Source: CAD feature listing. Evaluate the final solid. Frame: model axes, mm. Face numbers are marked on the shaded views. A direction names the side the tool comes from. Give positions to 0.01 mm unless a question says otherwise; leave off trailing zeros. Loops run counter-clockwise (first coordinate to the right, second up) from the corner with the lowest first, then second, coordinate; pieces in that order, holes last.
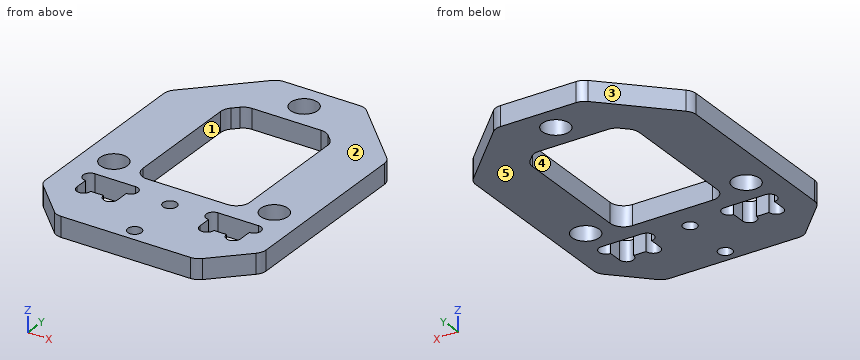
```python
from build123d import *

# Parameters (mm, degrees)
SKETCH_1_W          = 33
SKETCH_1_H          = 44.5
EXTRUDE_1_DEPTH     = 3
SKETCH_2_R          = 2.025
SKETCH_2_R_2        = 1.025
CUT_EXTRUDE_1_DEPTH = 13
CHAMFER_1_SIZE      = 10
CUT_EXTRUDE_2_DEPTH = 13
FILLET_1_R          = 2
CHAMFER_2_SIZE      = 6
FILLET_2_R          = 2
SKETCH_4_W          = 6.1
SKETCH_4_H          = 4.1
CUT_EXTRUDE_3_DEPTH = 3
SKETCH_5_R          = 1.05
CUT_EXTRUDE_4_DEPTH = 3


with BuildPart() as part:
    # 草图1 → 凸台-拉伸1 (new body)
    with BuildSketch(Plane.XY):
        Rectangle(SKETCH_1_W, SKETCH_1_H)
    extrude(amount=EXTRUDE_1_DEPTH)

    # 草图2 → 切除-拉伸1 (cut)
    with BuildSketch(Plane.XY.offset(3)):
        with Locations((12, -6.75)):
            Circle(SKETCH_2_R)
        with Locations((-12, -6.75)):
            Circle(SKETCH_2_R)
        with Locations((0, 18.25)):
            Circle(SKETCH_2_R)
        with Locations((0, -12.25)):
            Circle(SKETCH_2_R_2)
        with Locations((0, -20.25)):
            Circle(SKETCH_2_R_2)
    extrude(amount=-CUT_EXTRUDE_1_DEPTH, mode=Mode.SUBTRACT)

    # 倒角1
    chamfer_1_edges = [part.edges().sort_by_distance(p)[0] for p in [
        (-16.5, 22.25, 1.5),
        (16.5, 22.25, 1.5),
    ]]
    chamfer(chamfer_1_edges, length=CHAMFER_1_SIZE)

    # 草图3 → 切除-拉伸2 (cut)
    with BuildSketch(Plane.XY.offset(3)):
        Polygon((-8, -8.25), (8, -8.25), (8, 12.264718626), (6.014718626, 14.25), (-6.014718626, 14.25), (-8, 12.264718626), align=None)
    extrude(amount=-CUT_EXTRUDE_2_DEPTH, mode=Mode.SUBTRACT)

    # 圆角1
    fillet_1_edges = [part.edges().sort_by_distance(p)[0] for p in [
        (-8, -8.25, 1.5),
        (-8, 12.264718626, 1.5),
        (-6.014718626, 14.25, 1.5),
        (6.014718626, 14.25, 1.5),
        (8, 12.264718626, 1.5),
        (8, -8.25, 1.5),
    ]]
    fillet(fillet_1_edges, radius=FILLET_1_R)

    # 倒角2
    chamfer_2_edges = [part.edges().sort_by_distance(p)[0] for p in [
        (16.5, -22.25, 1.5),
        (-16.5, -22.25, 1.5),
    ]]
    chamfer(chamfer_2_edges, length=CHAMFER_2_SIZE)

    # 圆角2
    fillet_2_edges = [part.edges().sort_by_distance(p)[0] for p in [
        (16.5, -16.25, 1.5),
        (-10.5, -22.25, 1.5),
        (10.5, -22.25, 1.5),
        (-16.5, -16.25, 1.5),
        (-6.5, 22.25, 1.5),
        (6.5, 22.25, 1.5),
        (16.5, 12.25, 1.5),
        (-16.5, 12.25, 1.5),
    ]]
    fillet(fillet_2_edges, radius=FILLET_2_R)

    # 草图4 → 切除-拉伸3 (cut)
    with BuildSketch(Plane.XY.offset(3)):
        with Locations((-9.2, -12.75)):
            Rectangle(SKETCH_4_W, SKETCH_4_H)
        with Locations((9.2, -12.75)):
            Rectangle(SKETCH_4_W, SKETCH_4_H)
    extrude(amount=-CUT_EXTRUDE_3_DEPTH, mode=Mode.SUBTRACT)

    # 草图5 → 切除-拉伸4 (cut)
    with BuildSketch(Plane.XY.offset(3)):
        with Locations((-11.2, -14.8)):
            Circle(SKETCH_5_R)
        with Locations((-7.2, -14.8)):
            Circle(SKETCH_5_R)
        with Locations((7.2, -14.8)):
            Circle(SKETCH_5_R)
        with Locations((11.2, -14.8)):
            Circle(SKETCH_5_R)
        with Locations((-12.25, -11.75)):
            Circle(SKETCH_5_R)
        with Locations((-6.15, -11.75)):
            Circle(SKETCH_5_R)
        with Locations((6.15, -11.75)):
            Circle(SKETCH_5_R)
        with Locations((12.25, -11.75)):
            Circle(SKETCH_5_R)
    extrude(amount=-CUT_EXTRUDE_4_DEPTH, mode=Mode.SUBTRACT)


solid = part.part
```
(1) Section B-B, the plane y = -11.75. Return the cut outline in (x, z), then the cut area to 3 significant figures.
A:
outline: (-16.5, 0) - (-13.3, 0) - (-13.3, 3) - (-16.5, 3) - close; (-5.1, 0) - (-0.89, 0) - (-0.89, 3) - (-5.1, 3) - close; (0.89, 0) - (5.1, 0) - (5.1, 3) - (0.89, 3) - close; (13.3, 0) - (16.5, 0) - (16.5, 3) - (13.3, 3) - close
area: 44.4 mm2
(2) Mould query, pull axis Y, two halves, no side actions, for the marked faces 1, 2 and 3. Classes: pulls with the +Y half, pulls with the -Y half, needs draft (parallel to the pull), parting line crosses it, or undercut.
A:
face 1: undercut
face 2: needs draft
face 3: pulls with the +Y half
(3) Section D-D, the plane z = 1.7. Count the separate pieces of the cut face and the enclosed holes in it, then the cut area to 3 significant figures.
A:
separate pieces: 1
enclosed holes: 8
area: 869 mm2
(4) First-contact query: pin 1 (1 mm diameter, centred on y = -17.5, z = 2.5, fed in from -X); pin 2 (1.5 mm diameter, centred on x = 13, z = 2, fed in from +Y). Flat tips, straight axial feed; report the tip coordinate or a pass-through.
A:
pin 1: stops at x = -15.75
pin 2: stops at y = 16.5
(5) Reachability of the marked faces 4 and 5 from +Z, -Z, +X, -X, +Y, -Y: full face, straight path, thin tool, end or side. Return the list, or none.
A:
face 4: +Z, -Z
face 5: -Z, +X, -X, +Y, -Y
(6) Section C-C, the plane y = -20.25. Return the cut outline in (x, z) (3 decimals).
A:
outline: (-12.5, 0) - (-1.025, 0) - (-1.025, 3) - (-12.5, 3) - close; (1.025, 0) - (12.5, 0) - (12.5, 3) - (1.025, 3) - close
(7) Ray query, line 1 along Y through (x, z) = (0, 1.1) (3 decimals); line 2 along X through (y, z) = (16.5, 1.1); line 3 along X through (y, z) = (2, 2.3). Return the intervals inside material, ascending.
A:
line 1: y = -22.25 to -21.275, -19.225 to -13.275, -11.225 to -8.25, 14.25 to 16.225, 20.275 to 22.25
line 2: x = -12.25 to -1.02, 1.02 to 12.25
line 3: x = -16.5 to -8, 8 to 16.5
(8) Section A-A, the plane y = 18.25. Return the cut outline in (x, z) (3 decimals), then the cut area to 4 significant figures.
A:
outline: (-10.5, 0) - (-2.025, 0) - (-2.025, 3) - (-10.5, 3) - close; (2.025, 0) - (10.5, 0) - (10.5, 3) - (2.025, 3) - close
area: 50.85 mm2
